Work out the finished part from the listing and answer in its coordinate system (mm). A direction names the side the tool comes from. Round coordinates to 2 decimals unless told otherwise and drop trailing zeros. Order: outer loops, then holes, each group sorted by start corner. A loop starts at its lowest first (then second) coordinate and runs counter-clockwise, first axis right, second up. Notation, with made-up numbers: (-19.75, 44.25) - (-3.75, 44.25) arc R38 cw to (-3.75, 83.25) - close; hole circle Ø1 at (40, -12). An arc over 180 degrees is marked (long way). Put each result on its own line as item: value.
Autodesk Inventor part; units mm, degrees
ref_plane "YZ Plane" through (0, 0, 0) normal (1, 0, 0) x (0, 1, 0)
ref_plane "XZ Plane" through (0, 0, 0) normal (0, 1, 0) x (-1, 0, 0)
ref_plane "XY Plane" through (0, 0, 0) normal (0, 0, 1) x (1, 0, 0)
sketch "Sketch1" plane through (0, 0, 0) normal (0, 0, 1) x (1, 0, 0)
  circle A0 centre (0, 0) radius 9.7536
  line L0 (7.3323, 0) -> (3.6662, -6.35)
  line L1 (3.6662, -6.35) -> (-3.6662, -6.35)
  line L2 (-3.6662, -6.35) -> (-7.3323, 0)
  line L3 (-7.3323, 0) -> (-3.6662, 6.35)
  line L4 (-3.6662, 6.35) -> (3.6662, 6.35)
  line L5 (3.6662, 6.35) -> (7.3323, 0)
  dimension "d1" = 19.5072
  dimension "d2" = 12.7
extrude "Extrusion1" add sketch "Sketch1" along normal mid plane 12.6492
properties part number "0.498 Spacer 0.5 Hex"
1) Straight lines are drawn through the part: L1, parallel to Y at x = 0, z = 2; L2, parallel to X at y = -1.75, z = -5.5. For each, find the intervals that lie inside material, in ascending order. Write a range as from..to.
Findings below:
L1: y = -9.75..-6.35, 6.35..9.75
L2: x = -9.6..-6.32, 6.32..9.6
2) Given pin 1 Ø6 at (x, z) = (4.5, 3.5) entering from +Y; pin 2 Ø5 at (x, z) = (5.5, 0.5) entering from +Y; pin 3 Ø2 at (y, z) = (-5, -2.5) entering from +X, each flat-ended and moving along its own axis, determine where each tip first touches the part or whether it passes through.
Findings below:
pin 1: stops at y = 9.64
pin 2: stops at y = 9.28
pin 3: stops at x = 8.9
3) A cutting plane is placed at A-A on x = 0. Write down the section's boundary in (y, z).
Findings below:
outline: (-9.75, -6.32) - (-6.35, -6.32) - (-6.35, 6.32) - (-9.75, 6.32) - close; (6.35, -6.32) - (9.75, -6.32) - (9.75, 6.32) - (6.35, 6.32) - close
4) For a pull along Y with two mould halves and no side action, classify faces 1 (the flat face through (6.4, -2, -6.325)), 2 (the cylindrical face through (9.303, -2.93, -0.089)), 3 (the flat face through (5.474, 3.219, 0.089)), 4 (the flat face through (0, -6.35, 0)) as pulls with the +Y half, pulls with the -Y half, needs draft (parallel to the pull), parting line crosses it, or undercut.
Findings below:
face 1: needs draft
face 2: parting line crosses it
face 3: undercut
face 4: undercut
5) A cutting plane is placed at D-D on y = -7.5. Write down the section's boundary in (x, z), then the cut area to 3 significant figures.
Findings below:
outline: (-6.24, -6.32) - (6.24, -6.32) - (6.24, 6.32) - (-6.24, 6.32) - close
area: 158 mm2
6) For faces 5 (the flat face through (6.4, -2, 6.325)), 6 (the flat face through (-5.525, 3.131, 0.089)), determine the directions among +Z, -Z, +X, -X, +Y, -Y from which every point of the face is accessible in a straight line to the end or side of a thin tool.
Findings below:
face 5: +Z, +X, -X, +Y, -Y
face 6: +Z, -Z
7) A cutting plane is placed at C-C on y = -1. Write down the section's boundary in (x, z).
Findings below:
outline: (-9.7, -6.32) - (-6.75, -6.32) - (-6.75, 6.32) - (-9.7, 6.32) - close; (6.75, -6.32) - (9.7, -6.32) - (9.7, 6.32) - (6.75, 6.32) - close
8) A cutting plane is placed at B-B on z = -4.75. Write down the section's boundary in (x, y).
Findings below:
outline: circle Ø19.51 at (0, 0); hole (-7.33, 0) - (-3.67, -6.35) - (3.67, -6.35) - (7.33, 0) - (3.67, 6.35) - (-3.67, 6.35) - close
